```python
from build123d import *

# Parameters (mm, degrees)
AUFSATZ_LINEAR_AUSTRAGEN1_DEPTH = 3
SKIZZE2_R                       = 5
SKIZZE2_R_2                     = 3.2
SCHNITT_LINEAR_AUSTRAGEN1_DEPTH = 3
SKIZZE3_R                       = 3.2
SCHNITT_LINEAR_AUSTRAGEN2_DEPTH = 3
SKIZZE5_R                       = 1.6
SKIZZE5_R_2                     = 2.25
SCHNITT_LINEAR_AUSTRAGEN3_DEPTH = 3
SKIZZE7_R                       = 0.5
SCHNITT_LINEAR_AUSTRAGEN4_DEPTH = 110.64260121
VERRUNDUNG1_R                   = 10
ECSS_BEFESTIGUNG_DEPTH          = 110.64260121
SKIZZE9_R                       = 0.5
SCHNITT_LINEAR_AUSTRAGEN6_DEPTH = 110.64260121
KREISMUSTER1_COUNT              = 4
SKIZZE10_W                      = 4
SKIZZE10_H                      = 12
BEFESTIGUNG_SPANNTESTER_DEPTH   = 110.64260121
VERRUNDUNG2_R                   = 1
M4_GEWINDEBOHRUNG1_D            = 3.3
SKIZZE16_R                      = 0.5
SCHNITT_LINEAR_AUSTRAGEN8_DEPTH = 110.64260121
M4_GEWINDEBOHRUNG2_D            = 3.3


with BuildPart() as part:
    # Skizze1 → Aufsatz-Linear austragen1 (new body)
    with BuildSketch(Plane.XY):
        with BuildLine():
            Line((30, 54.748737342), (-30, 54.748737342))
            Line((-30, 54.748737342), (-47.625631329, 72.374368671))
            ThreePointArc((-47.625631329, 72.374368671), (-72.374368671, 72.374368671), (-72.374368671, 47.625631329))
            Line((-72.374368671, 47.625631329), (-49.748737342, 25))
            Line((-49.748737342, 25), (-60.45243751, -35.703700169))
            Line((-60.45243751, -35.703700169), (-72.374368671, -47.625631329))
            ThreePointArc((-72.374368671, -47.625631329), (-72.374368671, -72.374368671), (-47.625631329, -72.374368671))
            Line((-47.625631329, -72.374368671), (-30, -54.748737342))
            Line((-30, -54.748737342), (30, -54.748737342))
            Line((30, -54.748737342), (47.625631329, -72.374368671))
            ThreePointArc((47.625631329, -72.374368671), (72.374368671, -72.374368671), (72.374368671, -47.625631329))
            Line((72.374368671, -47.625631329), (60.45243751, -35.703700169))
            Line((60.45243751, -35.703700169), (49.748737342, 25))
            Line((49.748737342, 25), (72.374368671, 47.625631329))
            ThreePointArc((72.374368671, 47.625631329), (72.374368671, 72.374368671), (47.625631329, 72.374368671))
            Line((47.625631329, 72.374368671), (30, 54.748737342))
        make_face()
    extrude(amount=AUFSATZ_LINEAR_AUSTRAGEN1_DEPTH)

    # Skizze2 → Schnitt-Linear austragen1 (cut)
    with BuildSketch(Plane.XY.offset(3)):
        with Locations((-45.504310986, 45.504310986)):
            Circle(SKIZZE2_R)
        with Locations((-60, 60)):
            Circle(SKIZZE2_R_2)
        with Locations((45.504310986, 45.504310986)):
            Circle(SKIZZE2_R)
        with Locations((45.504310986, -45.504310986)):
            Circle(SKIZZE2_R)
        with Locations((-45.504310986, -45.504310986)):
            Circle(SKIZZE2_R)
        with Locations((-60, -60)):
            Circle(SKIZZE2_R_2)
        with Locations((60, 60)):
            Circle(SKIZZE2_R_2)
        with Locations((60, -60)):
            Circle(SKIZZE2_R_2)
    extrude(amount=-SCHNITT_LINEAR_AUSTRAGEN1_DEPTH, mode=Mode.SUBTRACT)

    # Skizze3 → Schnitt-Linear austragen2 (cut)
    with BuildSketch(Plane.XY.offset(3)):
        with Locations((-60, 60)):
            Circle(SKIZZE3_R)
        with BuildLine():
            ThreePointArc((65.303300859, 65.303300859), (65.303300859, 70.960155108), (70.960155108, 70.960155108))
            ThreePointArc((70.960155108, 70.960155108), (74.320132754, 54.068406798), (60, 44.5))
            ThreePointArc((60, 44.5), (56, 48.5), (60, 52.5))
            ThreePointArc((60, 52.5), (66.929096494, 57.129874257), (65.303300859, 65.303300859))
        make_face()
        with BuildLine():
            ThreePointArc((-70.960155108, 70.960155108), (-54.068406798, 74.320132754), (-44.5, 60))
            ThreePointArc((-44.5, 60), (-48.5, 56), (-52.5, 60))
            ThreePointArc((-52.5, 60), (-57.129874257, 66.929096494), (-65.303300859, 65.303300859))
            ThreePointArc((-65.303300859, 65.303300859), (-70.960155108, 65.303300859), (-70.960155108, 70.960155108))
        make_face()
        with BuildLine():
            ThreePointArc((65.303300859, -65.303300859), (57.129874257, -66.929096494), (52.5, -60))
            ThreePointArc((52.5, -60), (48.5, -56), (44.5, -60))
            ThreePointArc((44.5, -60), (54.068406798, -74.320132754), (70.960155108, -70.960155108))
            ThreePointArc((70.960155108, -70.960155108), (70.960155108, -65.303300859), (65.303300859, -65.303300859))
        make_face()
        with BuildLine():
            ThreePointArc((-70.960155108, -70.960155108), (-74.320132754, -54.068406798), (-60, -44.5))
            ThreePointArc((-60, -44.5), (-56, -48.5), (-60, -52.5))
            ThreePointArc((-60, -52.5), (-66.929096494, -57.129874257), (-65.303300859, -65.303300859))
            ThreePointArc((-65.303300859, -65.303300859), (-65.303300859, -70.960155108), (-70.960155108, -70.960155108))
        make_face()
    extrude(amount=-SCHNITT_LINEAR_AUSTRAGEN2_DEPTH, mode=Mode.SUBTRACT)

    # Skizze5 → Schnitt-Linear austragen3 (cut)
    with BuildSketch(Plane.XY.offset(3)):
        with Locations((-15.25, 15.25)):
            Circle(SKIZZE5_R)
        with Locations((15.25, 15.25)):
            Circle(SKIZZE5_R)
        with Locations((15.25, -15.25)):
            Circle(SKIZZE5_R)
        with Locations((-15.25, -15.25)):
            Circle(SKIZZE5_R)
        with Locations((-32.36, 13)):
            Circle(SKIZZE5_R_2)
        with Locations((-32.36, -13)):
            Circle(SKIZZE5_R_2)
        with BuildLine():
            Line((31.11, 15.25), (33.61, 15.25))
            ThreePointArc((33.61, 15.25), (35.86, 13), (33.61, 10.75))
            Line((33.61, 10.75), (31.11, 10.75))
            ThreePointArc((31.11, 10.75), (28.86, 13), (31.11, 15.25))
        make_face()
        with BuildLine():
            Line((31.11, -10.75), (33.61, -10.75))
            ThreePointArc((33.61, -10.75), (35.86, -13), (33.61, -15.25))
            Line((33.61, -15.25), (31.11, -15.25))
            ThreePointArc((31.11, -15.25), (28.86, -13), (31.11, -10.75))
        make_face()
    extrude(amount=-SCHNITT_LINEAR_AUSTRAGEN3_DEPTH, mode=Mode.SUBTRACT)

    # Skizze7 → Schnitt-Linear austragen4 (cut, through all)
    with BuildSketch(Plane.XY.offset(3)):
        with Locations((-45.748737342, 29.5)):
            Circle(SKIZZE7_R)
        with Locations((-45.748737342, -29.5)):
            Circle(SKIZZE7_R)
        with Locations((45.748737342, -29.5)):
            Circle(SKIZZE7_R)
        with Locations((45.748737342, 29.5)):
            Circle(SKIZZE7_R)
    extrude(amount=-SCHNITT_LINEAR_AUSTRAGEN4_DEPTH, mode=Mode.SUBTRACT)

    # Verrundung1
    verrundung1_edges = [part.edges().sort_by_distance(p)[0] for p in [
        (-30, 54.748737342, 1.5),
        (30, 54.748737342, 1.5),
        (49.748737342, 25, 1.5),
        (60.45243751, -35.703700169, 1.5),
        (30, -54.748737342, 1.5),
        (-30, -54.748737342, 1.5),
        (-60.45243751, -35.703700169, 1.5),
        (-49.748737342, 25, 1.5),
    ]]
    fillet(verrundung1_edges, radius=VERRUNDUNG1_R)

    # Skizze8 → ECSs Befestigung (cut, through all)
    with BuildSketch(Plane.XY.offset(3)):
        with BuildLine():
            Line((25.528544417, -38.256466479), (27.29631137, -40.024233431))
            ThreePointArc((27.29631137, -40.024233431), (27.29631137, -42.145553775), (25.174991027, -42.145553775))
            Line((25.174991027, -42.145553775), (23.407224074, -40.377786822))
            ThreePointArc((23.407224074, -40.377786822), (23.407224074, -38.256466479), (25.528544417, -38.256466479))
        make_face()
        with BuildLine():
            Line((38.610019869, -28.710524932), (36.842252916, -26.94275798))
            ThreePointArc((36.842252916, -26.94275798), (36.842252916, -24.821437636), (38.96357326, -24.821437636))
            Line((38.96357326, -24.821437636), (40.731340213, -26.589204589))
            ThreePointArc((40.731340213, -26.589204589), (40.731340213, -28.710524932), (38.610019869, -28.710524932))
        make_face()
        with BuildLine():
            Line((-38.610019869, -28.710524932), (-36.842252916, -26.94275798))
            ThreePointArc((-36.842252916, -26.94275798), (-36.842252916, -24.821437636), (-38.96357326, -24.821437636))
            Line((-38.96357326, -24.821437636), (-40.731340213, -26.589204589))
            ThreePointArc((-40.731340213, -26.589204589), (-40.731340213, -28.710524932), (-38.610019869, -28.710524932))
        make_face()
        with BuildLine():
            Line((-25.528544417, -38.256466479), (-27.29631137, -40.024233431))
            ThreePointArc((-27.29631137, -40.024233431), (-27.29631137, -42.145553775), (-25.174991027, -42.145553775))
            Line((-25.174991027, -42.145553775), (-23.407224074, -40.377786822))
            ThreePointArc((-23.407224074, -40.377786822), (-23.407224074, -38.256466479), (-25.528544417, -38.256466479))
        make_face()
        with BuildLine():
            Line((-25.528544417, 38.256466479), (-27.29631137, 40.024233431))
            ThreePointArc((-27.29631137, 40.024233431), (-27.29631137, 42.145553775), (-25.174991027, 42.145553775))
            Line((-25.174991027, 42.145553775), (-23.407224074, 40.377786822))
            ThreePointArc((-23.407224074, 40.377786822), (-23.407224074, 38.256466479), (-25.528544417, 38.256466479))
        make_face()
        with BuildLine():
            Line((-38.610019869, 28.710524932), (-36.842252916, 26.94275798))
            ThreePointArc((-36.842252916, 26.94275798), (-36.842252916, 24.821437636), (-38.96357326, 24.821437636))
            Line((-38.96357326, 24.821437636), (-40.731340213, 26.589204589))
            ThreePointArc((-40.731340213, 26.589204589), (-40.731340213, 28.710524932), (-38.610019869, 28.710524932))
        make_face()
        with BuildLine():
            Line((38.610019869, 28.710524932), (36.842252916, 26.94275798))
            ThreePointArc((36.842252916, 26.94275798), (36.842252916, 24.821437636), (38.96357326, 24.821437636))
            Line((38.96357326, 24.821437636), (40.731340213, 26.589204589))
            ThreePointArc((40.731340213, 26.589204589), (40.731340213, 28.710524932), (38.610019869, 28.710524932))
        make_face()
        with BuildLine():
            Line((25.528544417, 38.256466479), (27.29631137, 40.024233431))
            ThreePointArc((27.29631137, 40.024233431), (27.29631137, 42.145553775), (25.174991027, 42.145553775))
            Line((25.174991027, 42.145553775), (23.407224074, 40.377786822))
            ThreePointArc((23.407224074, 40.377786822), (23.407224074, 38.256466479), (25.528544417, 38.256466479))
        make_face()
    extrude(amount=-ECSS_BEFESTIGUNG_DEPTH, mode=Mode.SUBTRACT)

    # Skizze9 → Schnitt-Linear austragen6 (cut, through all)
    with BuildSketch(Plane.XY.offset(3)):
        with Locations((46.211417767, 62.474873734)):
            Circle(SKIZZE9_R)
    schnitt_linear_austragen6 = extrude(amount=-SCHNITT_LINEAR_AUSTRAGEN6_DEPTH, mode=Mode.SUBTRACT)

    # Kreismuster1: Schnitt-Linear austragen6 ×4 about axis
    kreismuster1_axis = Axis((0, 0, 0), (0, 0, 1))
    for i in range(1, KREISMUSTER1_COUNT):
        add(schnitt_linear_austragen6.rotate(kreismuster1_axis, i * 360 / KREISMUSTER1_COUNT), mode=Mode.SUBTRACT)

    # Skizze10 → Befestigung SpannTester (cut, through all)
    with BuildSketch(Plane.XY.offset(3)):
        with Locations((-16, -43.748737342)):
            Rectangle(SKIZZE10_W, SKIZZE10_H)
        with Locations((16, -43.748737342)):
            Rectangle(SKIZZE10_W, SKIZZE10_H)
    extrude(amount=-BEFESTIGUNG_SPANNTESTER_DEPTH, mode=Mode.SUBTRACT)

    # Verrundung2
    verrundung2_edges = [part.edges().sort_by_distance(p)[0] for p in [
        (-18, -49.748737342, 1.5),
        (-18, -37.748737342, 1.5),
        (-14, -37.748737342, 1.5),
        (-14, -49.748737342, 1.5),
        (18, -37.748737342, 1.5),
        (18, -49.748737342, 1.5),
        (14, -49.748737342, 1.5),
        (14, -37.748737342, 1.5),
    ]]
    fillet(verrundung2_edges, radius=VERRUNDUNG2_R)

    # M4 Gewindebohrung1 (through all)
    with Locations(Plane.XY.offset(3)):
        with Locations((-45.748737342, 29.5), (-62.474873734, 46.211417767), (-46.211417767, -62.474873734), (-45.748737342, -29.5), (45.748737342, 29.5), (45.748737342, -29.5), (62.474873734, -46.211417767), (46.211417767, 62.474873734)):
            Hole(M4_GEWINDEBOHRUNG1_D / 2)

    # Skizze16 → Schnitt-Linear austragen8 (cut, through all)
    with BuildSketch(Plane.XY.offset(3)):
        with Locations((-51.868272016, -68.131727984)):
            Circle(SKIZZE16_R)
        with Locations((-68.131727984, 51.868272016)):
            Circle(SKIZZE16_R)
        with Locations((51.868272016, 68.131727984)):
            Circle(SKIZZE16_R)
        with Locations((68.131727984, -51.868272016)):
            Circle(SKIZZE16_R)
    extrude(amount=-SCHNITT_LINEAR_AUSTRAGEN8_DEPTH, mode=Mode.SUBTRACT)

    # M4 Gewindebohrung2 (through all)
    with Locations(Plane.XY.offset(3)):
        with Locations((-51.868272016, -68.131727984), (-68.131727984, 51.868272016), (51.868272016, 68.131727984), (68.131727984, -51.868272016)):
            Hole(M4_GEWINDEBOHRUNG2_D / 2)


solid = part.part
```
Can you work these out from the model? Positions are in its coordinate system, mm. A direction names the side the tool comes from. Round coordinates to 2 decimals unless told otherwise and drop trailing zeros. Order: outer loops, then holes, each group sorted by start corner. A loop starts at its lowest first (then second) coordinate and runs counter-clockwise, first axis right, second up. Notation, with made-up numbers: (7.5, 79) -> (41.5, 79) arc R34 cw to (41.5, 115) -> close; hole circle Ø1 at (-15.75, -11). An arc over 180 degrees is marked (long way). Return JSON: item names as keys, results as strings. Group by question number.
1. Which directions (+Z, -Z, +X, -X, +Y, -Y) give clear straight access to the entire face, cutting with the end or side of a thin tool? Please do faces 3 (the face through (-55.214, -5.995, 1.479)), 4 (the face through (-54.305, 74.416, 1.521)).
2. If we section it at B-B, the plane z = 0.6: Count the separate pieces of the cut face and the enclosed holes in it, then the cut area to 3 significant figures.
3. Will these pins go through, and if not, where does the flat tip stop? pin 1 (0.8 mm diameter, centred on x = 32.5, z = 1.5, fed in from +Y); pin 2 (1 mm diameter, centred on y = 18.5, z = 1, fed in from -X); pin 3 (2 mm diameter, centred on x = 45.75, y = 29.5, fed in from +Z).
4. We'd pull the mould along Z, two halves only. Please class faces 1 (the face through (61.713, -47.675, 1.479)), 2 (the face through (-1, 1, 0)): released by +Z, released by -Z, zero draft, split by the parting line, or undercut.
5. If we section it at A-A, the plane x = 0.5: Write out the boundary of the cut face in (y, z).
6. I need wall thicknesses on line 1 (X direction, y = 58.5, z = 2.85); line 2 (X direction, y = 51, z = 1.4); line 3 (X direction, y = 58, z = 1.1). Which ranges of each line are inside material? Lowest first, please. Write a range as [from, to].
Output values:
{
 "1": {"face 3": "+Z, -Z, -X", "face 4": "+Z, -Z"},
 "2": {"separate pieces": "1", "enclosed holes": "42", "area": "14,200 mm²"},
 "3": {"pin 1": "y = 57.65", "pin 2": "x = -50.98", "pin 3": "through"},
 "4": {"face 1": "zero draft", "face 2": "released by -Z"},
 "5": {"outline": "(-54.75, 0) -> (54.75, 0) -> (54.75, 3) -> (-54.75, 3) -> close"},
 "6": {"line 1": "[-77.44, -62.83], [-57.17, -52.21], [-44.79, -33.75], [33.75, 57.17], [62.83, 67.35], [75.43, 77.44]", "line 2": "[-75.01, -69.53], [-66.73, 56.88], [72.62, 75.01]", "line 3": "[-77.39, -62.5], [-57.5, -51.96], [-45.04, -33.25], [33.25, 57.5], [62.5, 67.23], [75.37, 77.39]"}
}
